Work out the finished part from the listing and answer in its coordinate system (mm). A direction names the side the tool comes from. Coordinates: 2 decimals unless noted, no trailing zeros. Write each loop counter-clockwise with the first axis right and the second up, starting at its lowest first coordinate (ties: lowest second). Pieces come first, ordered by that corner, then holes. Notation, with made-up numbers: (83.5, 12.25) - (88.5, 12.25) arc R22 cw to (88.5, 26.25) - close; hole circle Ø11 at (18.5, 52). An arc over 180 degrees is marked (long way). Answer as a JSON object with one key per item and string values. Group by question number.
from build123d import *

# Parameters (mm, degrees)
BOSS_EXTRUDE1_START = 0.2
BOSS_EXTRUDE1_DEPTH = 9.6
BOSS_EXTRUDE2_START = -10
BOSS_EXTRUDE2_DEPTH = 30
MIRROR1_START       = 9.8
MIRROR1_DEPTH       = 30
MIRROR1_START_2     = 30.2
MIRROR1_2_DEPTH     = 9.6
MIRROR1_START_3     = 39.8
MIRROR1_3_DEPTH     = 10.2
MIRROR1_START_4     = -22.1
MIRROR1_4_OUTLINE_R = 2.085
MIRROR1_4_DEPTH     = 3


with BuildPart() as part:
    # Sketch1 → Boss-Extrude1 (new body)
    with BuildSketch(Plane(origin=(0, 0, 0), x_dir=(1, 0, 0), z_dir=(0, 1, 0)).offset(BOSS_EXTRUDE1_START)):
        with BuildLine():
            ThreePointArc((-24.36, 17.3), (-29.850614043, 0), (-24.36, -17.3))
            Line((-24.36, -17.3), (-6, -17.3))
            Line((-6, -17.3), (-6, -21.3))
            Line((-6, -21.3), (0, -21.3))
            Line((0, -21.3), (0, -17.3))
            ThreePointArc((0, -17.3), (17.3, 0), (0, 17.3))
            Line((0, 17.3), (0, 21.3))
            Line((0, 21.3), (-6, 21.3))
            Line((-6, 21.3), (-6, 17.3))
            Line((-6, 17.3), (-24.36, 17.3))
        make_face()
        with BuildLine():
            Line((0, -13.7), (-22.1, -13.7))
            Line((-22.1, -13.7), (-22.1, 13.7))
            Line((-22.1, 13.7), (0, 13.7))
            ThreePointArc((0, 13.7), (5.251022882, 12.653725091), (9.7, 9.674709298))
            Line((9.7, 9.674709298), (9.7, 5.4))
            Line((9.7, 5.4), (15.7, 0))
            Line((15.7, 0), (9.7, -5.4))
            Line((9.7, -5.4), (9.7, -9.674709298))
            ThreePointArc((9.7, -9.674709298), (5.251022882, -12.653725091), (0, -13.7))
        make_face(mode=Mode.SUBTRACT)
    extrude(amount=BOSS_EXTRUDE1_DEPTH)

    # Sketch1<3> → Boss-Extrude2 (add)
    with BuildSketch(Plane(origin=(0, 0, 0), x_dir=(1, 0, 0), z_dir=(0, 1, 0)).offset(BOSS_EXTRUDE2_START)):
        with BuildLine():
            Line((9.7, 14.324803664), (9.7, 9.674709298))
            ThreePointArc((9.7, 9.674709298), (12.261151879, 6.111804528), (13.564518925, 1.921932967))
            Line((13.564518925, 1.921932967), (15.7, 0))
            Line((15.7, 0), (13.564518925, -1.921932967))
            ThreePointArc((13.564518925, -1.921932967), (12.261151879, -6.111804528), (9.7, -9.674709298))
            Line((9.7, -9.674709298), (9.7, -14.324803664))
            ThreePointArc((9.7, -14.324803664), (17.3, 0), (9.7, 14.324803664))
        make_face()
        with BuildLine():
            Line((9.7, -5.4), (9.7, -9.674709298))
            ThreePointArc((9.7, -9.674709298), (12.261151879, -6.111804528), (13.564518925, -1.921932967))
            Line((13.564518925, -1.921932967), (9.7, -5.4))
        make_face()
        with BuildLine():
            ThreePointArc((13.564518925, 1.921932967), (12.261151879, 6.111804528), (9.7, 9.674709298))
            Line((9.7, 9.674709298), (9.7, 5.4))
            Line((9.7, 5.4), (13.564518925, 1.921932967))
        make_face()
    extrude(amount=BOSS_EXTRUDE2_DEPTH)

    # Mirror1: read off the stored shape, not the designer's step
    # Mirror1 outline → Mirror1 (add)
    with BuildSketch(Plane(origin=(0, 0, 0), x_dir=(1, 0, 0), z_dir=(0, 1, 0)).offset(MIRROR1_START)):
        with BuildLine():
            Line((-22.1, -17.3), (-22.1, 17.3))
            Line((-22.1, 17.3), (-24.36, 17.3))
            ThreePointArc((-24.36, 17.3), (-29.850614043, 0), (-24.36, -17.3))
            Line((-24.36, -17.3), (-22.1, -17.3))
        make_face()
        with BuildLine():
            Line((9.7, -5.4), (9.7, -14.324803664))
            ThreePointArc((9.7, -14.324803664), (17.3, 0), (9.7, 14.324803664))
            Line((9.7, 14.324803664), (9.7, 5.4))
            Line((9.7, 5.4), (15.7, 0))
            Line((15.7, 0), (9.7, -5.4))
        make_face()
    extrude(amount=MIRROR1_DEPTH)

    # Mirror1 2 outline → Mirror1 2 (add)
    with BuildSketch(Plane(origin=(0, 0, 0), x_dir=(1, 0, 0), z_dir=(0, 1, 0)).offset(MIRROR1_START_2)):
        with BuildLine():
            Line((0, -13.7), (-22.1, -13.7))
            Line((-22.1, -13.7), (-22.1, -17.3))
            Line((-22.1, -17.3), (-6, -17.3))
            Line((-6, -17.3), (-6, -21.3))
            Line((-6, -21.3), (0, -21.3))
            Line((0, -21.3), (0, -17.3))
            ThreePointArc((0, -17.3), (5.073011759, -16.539484626), (9.7, -14.324803664))
            Line((9.7, -14.324803664), (9.7, -9.674709298))
            ThreePointArc((9.7, -9.674709298), (5.251022882, -12.653725091), (0, -13.7))
        make_face()
        with BuildLine():
            Line((-22.1, 17.3), (-22.1, 13.7))
            Line((-22.1, 13.7), (0, 13.7))
            ThreePointArc((0, 13.7), (5.251022882, 12.653725091), (9.7, 9.674709298))
            Line((9.7, 9.674709298), (9.7, 14.324803664))
            ThreePointArc((9.7, 14.324803664), (5.073011759, 16.539484626), (0, 17.3))
            Line((0, 17.3), (0, 21.3))
            Line((0, 21.3), (-6, 21.3))
            Line((-6, 21.3), (-6, 17.3))
            Line((-6, 17.3), (-22.1, 17.3))
        make_face()
    extrude(amount=MIRROR1_2_DEPTH)

    # Mirror1 3 outline → Mirror1 3 (add)
    with BuildSketch(Plane(origin=(0, 0, 0), x_dir=(1, 0, 0), z_dir=(0, 1, 0)).offset(MIRROR1_START_3)):
        with BuildLine():
            Line((9.7, -5.4), (9.7, -14.324803664))
            ThreePointArc((9.7, -14.324803664), (17.3, 0), (9.7, 14.324803664))
            Line((9.7, 14.324803664), (9.7, 5.4))
            Line((9.7, 5.4), (15.7, 0))
            Line((15.7, 0), (9.7, -5.4))
        make_face()
    extrude(amount=MIRROR1_3_DEPTH)

    # Mirror1 4 outline → Mirror1 4 (add)
    with BuildSketch(Plane.YZ.offset(MIRROR1_START_4)):
        with Locations((5, 5.75)):
            Circle(MIRROR1_4_OUTLINE_R)
        with Locations((5, -5.75)):
            Circle(MIRROR1_4_OUTLINE_R)
        with Locations((35, 5.75)):
            Circle(MIRROR1_4_OUTLINE_R)
        with Locations((35, -5.75)):
            Circle(MIRROR1_4_OUTLINE_R)
    extrude(amount=MIRROR1_4_DEPTH)


solid = part.part
Q1. Consider L1, parallel to Y at x = 3, z = -15.5; L2, parallel to Z at x = -12.5, y = 6.5; L3, parallel to X at y = 38, z = -6.5. Determine where each line is inside the solid, lowest interval first. Write a range as from..to.
Q2. Flat-ended cylindrical pins translate along their axes: pin 1 Ø4 at (x, z) = (2, -15) entering from -Y; pin 2 Ø2 at (y, z) = (2.5, 19.5) entering from -X; pin 3 Ø10.5 at (x, y) = (-16, 37) entering from +Z. Find the tip coordinate at first contact, or state that the pin passes through.
Q3. Section C-C on x = 12.5 is taken. Determine the outline of the cut face in (y, z).
Q4. Section B-B on x = -3 is taken. Determine the outline of the cut face in (y, z).
Q5. A tool of negligible diameter and unlimited length cuts with its end or side. For faces 1 (the face through (0, 5, 19)), 2 (the face through (-11, 5, -13.7)), 3 (the face through (-6, 5, -19)), 4 (the face through (9.7, 20, 10)), 5 (the face through (0, 35, -19)), from which of +Z, -Z, +X, -X, +Y, -Y can it reach the whole face along a straight path? Write none if from no direction.
Q6. Section A-A on y = 31.5 is taken. Determine the outline of the cut face in (x, z), plus the area to 3 significant figures.
Q7. For a pull along Z with two mould halves and no side action, classify faces 6 (the face through (5.181, 34.933, -12.682)), 7 (the face through (-24, 0.2, 0)), 8 (the face through (9.7, 20, -10)), 9 (the face through (-29.85, 19.72, -0.26)) as +Z half, -Z half, draft (parallel to the pull), parting line (faces both ways), or undercut.
Q8. Section D-D on y = 5 is taken. Determine the outline of the cut face in (x, z) (3 decimals).
Numbers:
{
 "1": {"L1": "y = 0.2..9.8, 30.2..39.8", "L2": "z = -17.3..-13.7, 13.7..17.3", "L3": "x = -29.14..-22.1, 9.7..16.03"},
 "2": {"pin 1": "stops at y = 0.2", "pin 2": "stops at x = -6", "pin 3": "stops at z = 17.3"},
 "3": {"outline": "(-10, -11.96) - (50, -11.96) - (50, -2.88) - (-10, -2.88) - close; (-10, 2.88) - (50, 2.88) - (50, 11.96) - (-10, 11.96) - close"},
 "4": {"outline": "(0.2, -21.3) - (9.8, -21.3) - (9.8, -13.7) - (0.2, -13.7) - close; (0.2, 13.7) - (9.8, 13.7) - (9.8, 21.3) - (0.2, 21.3) - close; (30.2, -21.3) - (39.8, -21.3) - (39.8, -13.7) - (30.2, -13.7) - close; (30.2, 13.7) - (39.8, 13.7) - (39.8, 21.3) - (30.2, 21.3) - close"},
 "5": {"face 1": "+Z, +X, +Y, -Y", "face 2": "+Y, -Y", "face 3": "-Z, -X, +Y, -Y", "face 4": "none", "face 5": "-Z, +X, +Y, -Y"},
 "6": {"outline": "(-24.36, -17.3) - (-6, -17.3) - (-6, -21.3) - (0, -21.3) - (0, -17.3) arc R17.3 ccw to (0, 17.3) - (0, 21.3) - (-6, 21.3) - (-6, 17.3) - (-24.36, 17.3) arc R30 ccw to start; hole (-22.1, -13.7) - (0, -13.7) arc R13.7 ccw to (9.7, -9.67) - (9.7, -5.4) - (15.7, 0) - (9.7, 5.4) - (9.7, 9.67) arc R13.7 ccw to (0, 13.7) - (-22.1, 13.7) - close", "area": "611 mm²"},
 "7": {"face 6": "undercut", "face 7": "draft", "face 8": "undercut", "face 9": "parting line"},
 "8": {"outline": "(-24.36, -17.3) - (-6, -17.3) - (-6, -21.3) - (0, -21.3) - (0, -17.3) arc R17.3 ccw to (0, 17.3) - (0, 21.3) - (-6, 21.3) - (-6, 17.3) - (-24.36, 17.3) arc R30 ccw to start; hole (-22.1, -13.7) - (0, -13.7) arc R13.7 ccw to (9.7, -9.675) - (9.7, -5.4) - (15.7, 0) - (9.7, 5.4) - (9.7, 9.675) arc R13.7 ccw to (0, 13.7) - (-22.1, 13.7) - (-22.1, 7.835) - (-19.1, 7.835) - (-19.1, 3.665) - (-22.1, 3.665) - (-22.1, -3.665) - (-19.1, -3.665) - (-19.1, -7.835) - (-22.1, -7.835) - close"}
}
